Autodesk Inventor part; units mm, degrees
ref_plane "YZ Plane" through (0, 0, 0) normal (1, 0, 0) x (0, 1, 0)
ref_plane "XZ Plane" through (0, 0, 0) normal (0, 1, 0) x (-1, 0, 0)
ref_plane "XY Plane" through (0, 0, 0) normal (0, 0, 1) x (1, 0, 0)
sketch "Sketch1" plane through (0, 0, 0) normal (0, 1, 0) x (-1, 0, 0)
  circle A0 centre (0, 0) radius 135
  circle A1 centre (0, 0) radius 110
  dimension "d0" = 270
  dimension "d1" = 220
extrude "Extrusion1" add sketch "Sketch1" along normal mid plane 20
sketch "Sketch2" plane through (0, 10, 0) normal (0, 1, 0) x (1, 0, 0)
  circle A0 centre (0, 0) radius 37.5
  circle A1 centre (0, 0) radius 135
  dimension "d4" = 75
  dimension "d20" = 270
extrude "Extrusion2" add sketch "Sketch2" against normal blind 1
sketch "Sketch3" plane through (0, 10, 0) normal (0, 1, 0) x (1, 0, 0)
  circle A0 centre (0, 0) radius 127.5
  circle A1 centre (127.5, 0) radius 2.5
  circle A2 centre (103.1497, 74.9426) radius 2.5
  circle A3 centre (39.3997, 121.2597) radius 2.5
  circle A4 centre (-39.3997, 121.2597) radius 2.5
  circle A5 centre (-103.1497, 74.9426) radius 2.5
  circle A6 centre (-127.5, 0) radius 2.5
  circle A7 centre (-103.1497, -74.9426) radius 2.5
  circle A8 centre (-39.3997, -121.2597) radius 2.5
  circle A9 centre (39.3997, -121.2597) radius 2.5
  circle A10 centre (103.1497, -74.9426) radius 2.5
  dimension "d7" = 255
  dimension "d8" = 5
  dimension "d11" = 360
hole "Hole1" at (127.5, 10, 0) at (103.1497, 10, 74.9426) at (39.3997, 10, 121.2597) at (-39.3997, 10, 121.2597) at (-103.1497, 10, 74.9426) at (-127.5, 10, 0) at (-103.1497, 10, -74.9426) at (-39.3997, 10, -121.2597) at (39.3997, 10, -121.2597) at (103.1497, 10, -74.9426) direction (0, -1, 0) diameter 5 end through all
properties part number "Cylinder Spacer 25mm"
Geometry: final body of the model. Coordinates: model frame, mm. Give positions to 0.01 mm unless a question says otherwise; leave off trailing zeros. Write each loop counter-clockwise with the first axis right and the second up, starting at its lowest first coordinate (ties: lowest second). Pieces come first, ordered by that corner, then holes.
1. Line query: probe 1 along Z at (x, y) = (0, -5); probe 2 along X at (y, z) = (1, 73.5); probe 3 along Y at (x, z) = (-32.5, -50). Output: solid intervals per line, ascending.
2. Section query C-C, the plane x = -81.5. Return loops of the section in (y, z).
3. Section query A-A, the plane x = 0. Return loops of the section in (y, z).
4. Draft query along Z for faces 1 (the flat face through (-2, 9, 47)), 2 (the cylindrical face through (107.13, -0.14, 82.15)), 3 (the cylindrical face through (23.846, -0.633, 107.384)), 4 (the flat face through (-28, 10, -28)). Return one class per face: released by +Z, released by -Z, zero draft, split by the parting line, or undercut.
5. Section query D-D, the plane y = 4.75. Count the separate pieces of the cut face and the enclosed holes in it, then the cut area to 3 significant figures.
6. Section query B-B, the plane z = 25. Return loops of the section in (x, y) (3 decimals), then the cut area to 3 significant figures.
7. Pin query (flat end, axial travel): P1, Ø4.5, axis at x = -127.5, z = 0, coming from the +Y side; P2, Ø5, axis at y = -5, z = -99.5, coming from the +X side; P3, Ø8, axis at x = -64, z = 34, coming from the -Y side; P4, Ø8, axis at x = -45.5, y = -2, coming from the +Z side. Return the tip coordinate at first contact, or that it passes through.
Computed:
1. probe 1: z = -135 to -110, 110 to 135
1. probe 2: x = -113.24 to -105.19, -101.11 to -81.84, 81.84 to 101.11, 105.19 to 113.24
1. probe 3: y = 9 to 10
2. outline: (-10, -107.62) - (10, -107.62) - (10, 107.62) - (-10, 107.62) - (-10, 73.88) - (9, 73.88) - (9, -73.88) - (-10, -73.88) - close
3. outline: (-10, -135) - (10, -135) - (10, -37.5) - (9, -37.5) - (9, -110) - (-10, -110) - close; (-10, 110) - (9, 110) - (9, 37.5) - (10, 37.5) - (10, 135) - (-10, 135) - close
4. face 1: undercut
4. face 2: split by the parting line
4. face 3: undercut
4. face 4: zero draft
5. separate pieces: 1
5. enclosed holes: 11
5. area: 19,000 mm2
6. outline: (-132.665, -10) - (-107.121, -10) - (-107.121, 9) - (-27.951, 9) - (-27.951, 10) - (-132.665, 10) - close; (27.951, 9) - (107.121, 9) - (107.121, -10) - (132.665, -10) - (132.665, 10) - (27.951, 10) - close
6. area: 1,180 mm2
7. P1: passes through
7. P2: stops at x = 93.89
7. P3: stops at y = 9
7. P4: stops at z = 128.46
